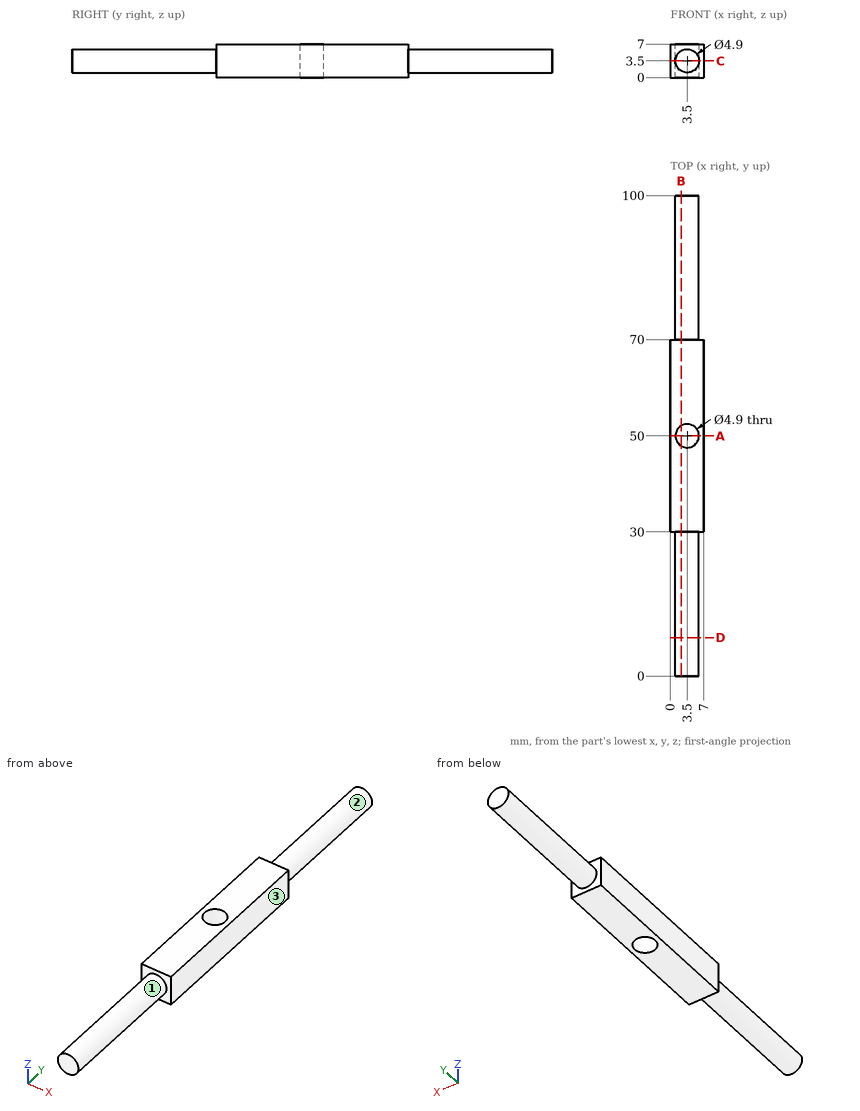
For this review, use the dimensioned drawing (mm, ordinates from the lowest corner) and the shaded views. A direction names the side the tool comes from. Coordinates: 2 decimals unless noted, no trailing zeros. Loops run counter-clockwise (first coordinate to the right, second up) from the corner with the lowest first, then second, coordinate; pieces in that order, holes last.
1. Add section B-B, the plane x = 2.25. Give the boundary of the cut face in (y, z), then the cut area to 3 significant figures.
2. Add section D-D, the plane y = 8. Give the boundary of the cut face in (x, z), then the cut area to 3 significant figures.
3. Insertion check: P1, Ø1.5, axis at x = 3.5, y = 27.5, coming from the +Z side. The pin has a flat end and moves straight along its axis. Give the tip position at first contact, or say it passes through.
4. For line 1 (Y direction, x = 3.5, z = 1.5); line 2 (Y direction, x = 2.75, z = 5); line 3 (Z direction, x = 3.75, y = 82), list the stretches that pass through material, from the lowest coordinate up.
5. Add section A-A, the plane y = 50. Give the boundary of the cut face in (x, z).
6. For the marked faces 1, 2 and 3, list the 3-axis set-ups (+Z, -Z, +X, -X, +Y, -Y) from which the entire face can be reached by the end or side of a thin tool; tool diameter is ignored.
7. Add section C-C, the plane z = 3.5. Give the boundary of the cut face in (x, y).
Result:
1. outline: (0, 1.39) - (30, 1.39) - (30, 0) - (47.89, 0) - (47.89, 7) - (30, 7) - (30, 5.61) - (0, 5.61) - close; (52.11, 0) - (70, 0) - (70, 1.39) - (100, 1.39) - (100, 5.61) - (70, 5.61) - (70, 7) - (52.11, 7) - close
1. area: 503 mm2
2. outline: circle Ø4.9 at (3.5, 3.5)
2. area: 18.9 mm2
3. P1: stops at z = 5.95
4. line 1: y = 0 to 47.55, 52.45 to 100
4. line 2: y = 0 to 47.67, 52.33 to 100
4. line 3: z = 1.06 to 5.94
5. outline: (0, 0) - (1.05, 0) - (1.05, 7) - (0, 7) - close; (5.95, 0) - (7, 0) - (7, 7) - (5.95, 7) - close
6. face 1: -Y
6. face 2: +Y
6. face 3: +Z, -Z, +X, +Y, -Y
7. outline: (0, 30) - (1.05, 30) - (1.05, 0) - (5.95, 0) - (5.95, 30) - (7, 30) - (7, 70) - (5.95, 70) - (5.95, 100) - (1.05, 100) - (1.05, 70) - (0, 70) - close; hole circle Ø4.9 at (3.5, 50)
